Could you check a few things on this model? Use its own coordinates, in mm. A direction names the side the tool comes from. Give positions to 0.01 mm unless a question says otherwise; leave off trailing zeros. Loops run counter-clockwise (first coordinate to the right, second up) from the corner with the lowest first, then second, coordinate; pieces in that order, holes last. Notation, with made-up numbers: M 40,-28.75 L 72,-28.75 A25 ccw 72,2.25 Z; hole C 73,55.5 d5. An arc over 180 degrees is marked long. Use a Markdown table: item, result. Add a question column.
1) Will these pins go through, and if not, where does the flat tip stop? pin 1 Ø5 at (x, z) = (1.5, -3) entering from -Y; pin 2 Ø1.1 at (x, z) = (8.5, -3) entering from -Y; pin 3 Ø2.5 at (y, z) = (6, 0) entering from -X.
2) Which directions (+Z, -Z, +X, -X, +Y, -Y) give clear straight access to the entire face, cutting with the end or side of a thin tool? Please do faces 4 (the flat face through (7, -3, 0)), 5 (the cylindrical face through (0.5, 7.2, -0.9)), 6 (the flat face through (5.5, 3.4, -1.7)).
3) Suppose I cut it at C-C on x = 8.25. List the corners of the cut face in (y, z) for me, and give its area (3 significant figures).
4) Suppose I cut it at A-A on y = 1. List the corners of the cut face in (x, z) for me, and give its area (3 significant figures).
5) We'd pull the mould along Z, two halves only. Please class faces 1 (the cylindrical face through (0.5, -4.8, -0.9)), 2 (the cylindrical face through (2.71, -1.73, -7.81)), 3 (the flat face through (8, 0, 3)): +Z half, -Z half, draft (parallel to the pull), parting line (faces both ways), or undercut.
6) Suppose I cut it at D-D on z = 1.75. List the corners of the cut face in (x, y) for me.
7) Suppose I cut it at B-B on x = 4. List the corners of the cut face in (y, z) for me, and give its area (3 significant figures).
8) If I drill on line 1 along X through (y, z) = (-0.5, 4); line 2 along Z through (x, y) = (4, 6); line 3 along Z through (x, y) = (6.5, 1.75), over which ranges is the centre line in solid material (lowest first)? Write a range as [from, to].
```python
from build123d import *
from build123d import SkipClean  # not in build123d's __all__

# Parameters (mm, degrees)
F0_R            = 8
F1_DEPTH        = 5.5
F2_R            = 3.5
F3_DEPTH        = 1.5
F5_DEPTH        = 2.5
F7_DEPTH        = 1.5
F9_D            = 3
F10_R           = 1.5
F11_DEPTH       = 1
F13_D           = 2
F13_CSINK_D     = 3
F13_CSINK_ANGLE = 90


with BuildPart() as f1:
    # F0 (on Right) → F1 (new body)
    with BuildSketch(Plane.YZ):
        Circle(F0_R)
    extrude(amount=F1_DEPTH)

    # F2 (on face) → F3 (join)
    with BuildSketch(Plane.YZ.offset(5.5)):
        Circle(F2_R)
    extrude(amount=F3_DEPTH)

    # F4 (on face) → F5 (join)
    with BuildSketch(Plane.YZ.offset(7)):
        with BuildLine():
            Line((0, -2.5), (0, -3.5))
            ThreePointArc((0, -3.5), (2.4748737342, -2.4748737342), (3.5, 0))
            ThreePointArc((3.5, 0), (2.4748737342, 2.4748737342), (0, 3.5))
            Line((0, 3.5), (0, 2.5))
            ThreePointArc((0, 2.5), (2.5, 0), (0, -2.5))
        make_face()
    extrude(amount=F5_DEPTH)

    # F6 (on face) → F7 (cut)
    with BuildSketch(Plane.YZ.offset(7)):
        with BuildLine():
            ThreePointArc((0, -2.5), (1.767766953, -1.767766953), (2.5, 0))
            ThreePointArc((2.5, 0), (1.767766953, 1.767766953), (0, 2.5))
            ThreePointArc((0, 2.5), (-2.5, 0), (0, -2.5))
        make_face()
    with SkipClean():  # cleaning this boolean's faces spoils the solid; the shape is the same uncleaned
        extrude(amount=-F7_DEPTH, mode=Mode.SUBTRACT)

    # F9 (through all)
    with Locations(Plane.YZ.offset(5.5)):
        with Locations((0, 0)):
            Hole(F9_D / 2)

    # F10 (on face) → F11 (cut)
    with BuildSketch(Plane(origin=(0, 0, 0), x_dir=(0, -1, 0), z_dir=(-1, 0, 0))):
        with Locations((-6, 0)):
            Circle(F10_R)
        with Locations((6, 0)):
            Circle(F10_R)
    extrude(amount=-F11_DEPTH, mode=Mode.SUBTRACT)

    # F13 (through all)
    with Locations(Plane(origin=(1, 0, 0), x_dir=(0, -1, 0), z_dir=(-1, 0, 0))):
        with Locations((-6, 0), (6, 0)):
            CounterSinkHole(F13_D / 2, F13_CSINK_D / 2, counter_sink_angle=F13_CSINK_ANGLE)


solid = f1.part
```
Answer block:
| question | item | result |
|---|---|---|
| 1 | pin 1 | stops at y = -7.98 |
| 1 | pin 2 | stops at y = 0 |
| 1 | pin 3 | stops at x = 1.25 |
| 2 | face 4 | +Z, -Z, +X, -Y |
| 2 | face 5 | -X |
| 2 | face 6 | +X |
| 3 | outline | M 0,-3.5 A3.5 ccw 0,3.5 L 0,2.5 A2.5 cw 0,-2.5 Z |
| 3 | area | 9.42 mm^2 |
| 4 | outline | M 0,-7.94 L 5.5,-7.94 L 5.5,-3.35 L 9.5,-3.35 L 9.5,-2.29 L 5.5,-2.29 L 5.5,-1.12 L 0,-1.12 Z; M 0,1.12 L 5.5,1.12 L 5.5,2.29 L 9.5,2.29 L 9.5,3.35 L 5.5,3.35 L 5.5,7.94 L 0,7.94 Z |
| 4 | area | 83.5 mm^2 |
| 5 | face 1 | undercut |
| 5 | face 2 | parting line |
| 5 | face 3 | draft |
| 6 | outline | M 0,-7.81 L 5.5,-7.81 L 5.5,-3.03 L 7,-3.03 L 7,-1.79 L 5.5,-1.79 L 5.5,1.79 L 9.5,1.79 L 9.5,3.03 L 5.5,3.03 L 5.5,7.81 L 0,7.81 Z |
| 7 | outline | C 0,0 d16; hole C -6,0 d2; hole C 0,0 d3; hole C 6,0 d2 |
| 7 | area | 188 mm^2 |
| 8 | line 1 | x = [0, 5.5] |
| 8 | line 2 | z = [-5.29, -1], [1, 5.29] |
| 8 | line 3 | z = [-3.03, -1.79], [1.79, 3.03] |
